Geometry check sheet. Reference: the model listing, model coordinates, mm. A direction names the side the tool comes from. Round coordinates to 2 decimals unless told otherwise and drop trailing zeros. Write each loop counter-clockwise with the first axis right and the second up, starting at its lowest first coordinate (ties: lowest second). Pieces come first, ordered by that corner, then holes. Notation, with made-up numbers: M 14,61.25 L 47,61.25 A26 ccw 47,100.25 Z; hole C 55,-16.5 d10. An arc over 180 degrees is marked long. Put each result on its own line as item: value. Start each with the question number.
(1) Section check D-D on x = 5. Record the cut outline in (y, z).
(2) Section check A-A on x = 19. Record the cut outline in (y, z).
(3) Section check B-B on y = -33. Record the cut outline in (x, z).
(4) Section check C-C on z = 50. Record the cut outline in (x, y).
(5) Tool access check on faces 1 (the flat face through (16.516, -38, 45)), 2 (the flat face through (0, -20.066, 17)), 3 (the flat face through (-27.08, -32.94, 54.79)). Record the directions out of +Z, -Z, +X, -X, +Y, -Y that give a thin tool (end or side, any length) a straight path to the whole face; none if there is none.
(6) Material ranges on probe 1 along X at (y, z) = (-30, 41); probe 2 along Y at (x, z) = (-23, 29); probe 3 along Z at (x, y) = (11, -43), recorded low to high.
(7) Gauge pin test, flat ends, axial feed: pin 1 (10 mm diameter, centred on x = -22.5, y = -28.5, fed in from -Z); pin 2 (12 mm diameter, centred on y = -40.5, z = 32.5, fed in from -X); pin 3 (8 mm diameter, centred on x = -27.5, z = 34, fed in from -Y). Record the tip position at first contact, or that the pin passes through.
from build123d import *

# Parameters (mm, degrees)
F1_DEPTH = 20.066
F0_W     = 23.2850266621
F0_H     = 43.0419966578
F0_W_2   = 23.8309800625
F2_DEPTH = 45.466
F4_DEPTH = 78.9115072618
F0_W_3   = 31.7945005372
F5_DEPTH = 45.466


with BuildPart() as f1:
    # F0 (on Front) → F1 (new body)
    with BuildSketch(Plane.XZ):
        Polygon((-38.5636128485, 32.9706594348), (-38.5636128485, 0), (40.3468944132, 0), (40.3468944132, 32.9706594348), (16.5159143507, 32.9706594348), (-15.2785861865, 32.9706594348), align=None)
    extrude(amount=F1_DEPTH)

    # F0 (on Front) → F2 (join)
    with BuildSketch(Plane.XZ):
        with Locations((-26.9210995175, 54.4916577637)):
            Rectangle(F0_W, F0_H)
        with Locations((28.431404382, 54.4916577637)):
            Rectangle(F0_W_2, F0_H)
    extrude(amount=F2_DEPTH)

    # F3 (on face) → F4 (cut, through all)
    with BuildSketch(Plane(origin=(-38.5636128485, 0, 0), x_dir=(0, -1, 0), z_dir=(-1, 0, 0))):
        Polygon((45.466, 32.9706594348), (45.466, 76.0126560926), (20.066, 32.9706594348), align=None)
    extrude(amount=-F4_DEPTH, mode=Mode.SUBTRACT)

    # F0 (on Front) → F5 (join)
    with BuildSketch(Plane.XZ):
        with Locations((0.6186640821, 54.4916577637)):
            Rectangle(F0_W_3, F0_H)
    extrude(amount=F5_DEPTH)


solid = f1.part
Answers follow:
1. outline: M -45.47,32.97 L -20.07,32.97 L -20.07,0 L 0,0 L 0,76.01 L -45.47,76.01 Z
2. outline: M -45.47,76.01 L -20.07,32.97 L -20.07,0 L 0,0 L 0,76.01 Z
3. outline: M -38.56,54.89 L -15.28,54.89 L -15.28,32.97 L 16.52,32.97 L 16.52,54.89 L 40.35,54.89 L 40.35,76.01 L -38.56,76.01 Z
4. outline: M -38.56,-30.12 L -15.28,-30.12 L -15.28,-45.47 L 16.52,-45.47 L 16.52,-30.12 L 40.35,-30.12 L 40.35,0 L -38.56,0 Z
5. face 1: -Z, +X, -Y
5. face 2: -Z, +X, -X, -Y
5. face 3: -Z, -X, -Y
6. probe 1: x = -15.28 to 16.52
6. probe 2: y = -20.07 to 0
6. probe 3: z = 32.97 to 76.01
7. pin 1: stops at z = 38.79
7. pin 2: stops at x = -15.28
7. pin 3: stops at y = -23.03
